The listing builds one solid part. Answer for the finished solid, in the listing's coordinates (mm). A direction names the side the tool comes from. Give positions to 0.01 mm unless a question says otherwise; leave off trailing zeros. Order: outer loops, then holes, each group sorted by start corner. A loop starts at its lowest first (then second) coordinate and runs counter-clockwise, first axis right, second up. Notation, with made-up numbers: (-13, 28) - (-6, 28) arc R17 cw to (-6, 49) - close; hole circle Ø9 at (3, 86.25). An arc over 180 degrees is marked (long way). Use CSV: the item, a comma, the result in double quotes.
```python
from build123d import *

# Parameters (mm, degrees)
RIGHT_PLATE_DEPTH         = 6.35
SKETCH5_R                 = 6.0325
SPOOL_POST_DEPTH          = 7.62
F_8_CLEARANCE_HOLE1_D     = 4.9149
F_8_CLEARANCE_HOLE1_DEPTH = 6.35
O_0_316_DIAMETER_HOLE3_D  = 8.0264


with BuildPart() as part:
    # Sketch1 → Right plate (new body)
    with BuildSketch(Plane(origin=(0, 0, 0), x_dir=(0, 0, -1), z_dir=(1, 0, 0))):
        with BuildLine():
            Line((-31.75, -50.8), (31.75, -50.8))
            ThreePointArc((31.75, -50.8), (36.240128061, -48.940128061), (38.1, -44.45))
            Line((38.1, -44.45), (38.1, 105.41))
            ThreePointArc((38.1, 105.41), (36.240128061, 109.900128061), (31.75, 111.76))
            Line((31.75, 111.76), (-31.75, 111.76))
            ThreePointArc((-31.75, 111.76), (-36.240128061, 109.900128061), (-38.1, 105.41))
            Line((-38.1, 105.41), (-38.1, -44.45))
            ThreePointArc((-38.1, -44.45), (-36.240128061, -48.940128061), (-31.75, -50.8))
        make_face()
    extrude(amount=RIGHT_PLATE_DEPTH)

    # Sketch5 → Spool post (add)
    with BuildSketch(Plane(origin=(6.35, 0, 0), x_dir=(0, 0, -1), z_dir=(1, 0, 0))):
        Circle(SKETCH5_R)
    extrude(amount=SPOOL_POST_DEPTH)

    # #8 Clearance Hole1
    with Locations(Plane.ZY):
        with Locations((-26.646533, 101.600261), (27.342012, 101.600261), (27.342012, 30.480261), (-26.646533, 30.480261), (-26.646533, -40.639739), (27.342012, -40.639739)):
            Hole(F_8_CLEARANCE_HOLE1_D / 2, depth=F_8_CLEARANCE_HOLE1_DEPTH)

    # O (0.316) Diameter Hole3 (through all)
    with Locations(Plane(origin=(6.35, 0, 0), x_dir=(0, 0, -1), z_dir=(1, 0, 0))):
        with Locations((-675.189894138, -31.321376827), (0, 50.8)):
            Hole(O_0_316_DIAMETER_HOLE3_D / 2)


solid = part.part
```
Item 1: The part is cut by section D-D (x = 1.5). Give the vertices of the cut face in (y, z).
Taken from the geometry:
outline,"(-50.8, -31.75) arc R6.35 ccw to (-44.45, -38.1) - (105.41, -38.1) arc R6.35 ccw to (111.76, -31.75) - (111.76, 31.75) arc R6.35 ccw to (105.41, 38.1) - (-44.45, 38.1) arc R6.35 ccw to (-50.8, 31.75) - close; hole circle Ø4.91 at (-40.64, -26.65); hole circle Ø4.91 at (-40.64, 27.34); hole circle Ø4.91 at (30.48, -26.65); hole circle Ø4.91 at (30.48, 27.34); hole circle Ø8.03 at (50.8, 0); hole circle Ø4.91 at (101.6, -26.65); hole circle Ø4.91 at (101.6, 27.34)"
Item 2: Which of the six approach directions +Z, -Z, +X, -X, +Y, -Y give full straight-line access (tool end or side, diameter ignored) to faces 1 (the face through (10.107, 1.812, -5.754)), 2 (the face through (3, -50.8, 0))?
Taken from the geometry:
face 1,"+X"
face 2,"+Z, -Z, +X, -X, -Y"
Item 3: Each of these flat-tipped pins is pushed along its axis until it touches: pin 1 (12 mm diameter, centred on y = 59.5, z = 17, fed in from +X); pin 2 (6 mm diameter, centred on x = 10.5, y = 1, fed in from -Z). Where does it stop, or does it pass through?
Taken from the geometry:
pin 1,"x = 6.35"
pin 2,"z = -6.03"
Item 4: The part is cut by section C-C (y = 0). Give the vertices of the cut face in (x, z), and give its area (3 significant figures).
Taken from the geometry:
outline,"(0, -38.1) - (6.35, -38.1) - (6.35, -6.03) - (13.97, -6.03) - (13.97, 6.03) - (6.35, 6.03) - (6.35, 38.1) - (0, 38.1) - close"
area,"576 mm^2"
Item 5: The mould has two halves that part along Z. Classify faces 3 (the face through (3.13, -48.89, 36.29)), 4 (the face through (0, 32, 1)), 5 (the face through (3.219, -43.039, -26.114)), 6 (the face through (3.13, 109.85, -36.29)): +Z half, -Z half, draft (parallel to the pull), parting line (faces both ways), or undercut.
Taken from the geometry:
face 3,"+Z half"
face 4,"draft"
face 5,"undercut"
face 6,"-Z half"
Item 6: The part is cut by section B-B (z = 0). Give the vertices of the cut face in (x, y), and give its area (3 significant figures).
Taken from the geometry:
outline,"(0, -50.8) - (6.35, -50.8) - (6.35, -6.03) - (13.97, -6.03) - (13.97, 6.03) - (6.35, 6.03) - (6.35, 46.79) - (0, 46.79) - close; (0, 54.81) - (6.35, 54.81) - (6.35, 111.76) - (0, 111.76) - close"
area,"1,070 mm^2"
Item 7: The part is cut by section A-A (y = 50.8). Give the vertices of the cut face in (x, z), and give its area (3 significant figures).
Taken from the geometry:
outline,"(0, -38.1) - (6.35, -38.1) - (6.35, -4.01) - (0, -4.01) - close; (0, 4.01) - (6.35, 4.01) - (6.35, 38.1) - (0, 38.1) - close"
area,"433 mm^2"
Item 8: Find the intervals of material crossed by line 1 along Y through (x, z) = (5, -26); line 2 along Y through (x, z) = (2, 0); line 3 along X through (y, z) = (63, -6), in increasing order.
Taken from the geometry:
line 1,"-50.8 to -43.01, -38.27 to 28.11, 32.85 to 99.23, 103.97 to 111.76"
line 2,"-50.8 to 46.79, 54.81 to 111.76"
line 3,"0 to 6.35"
